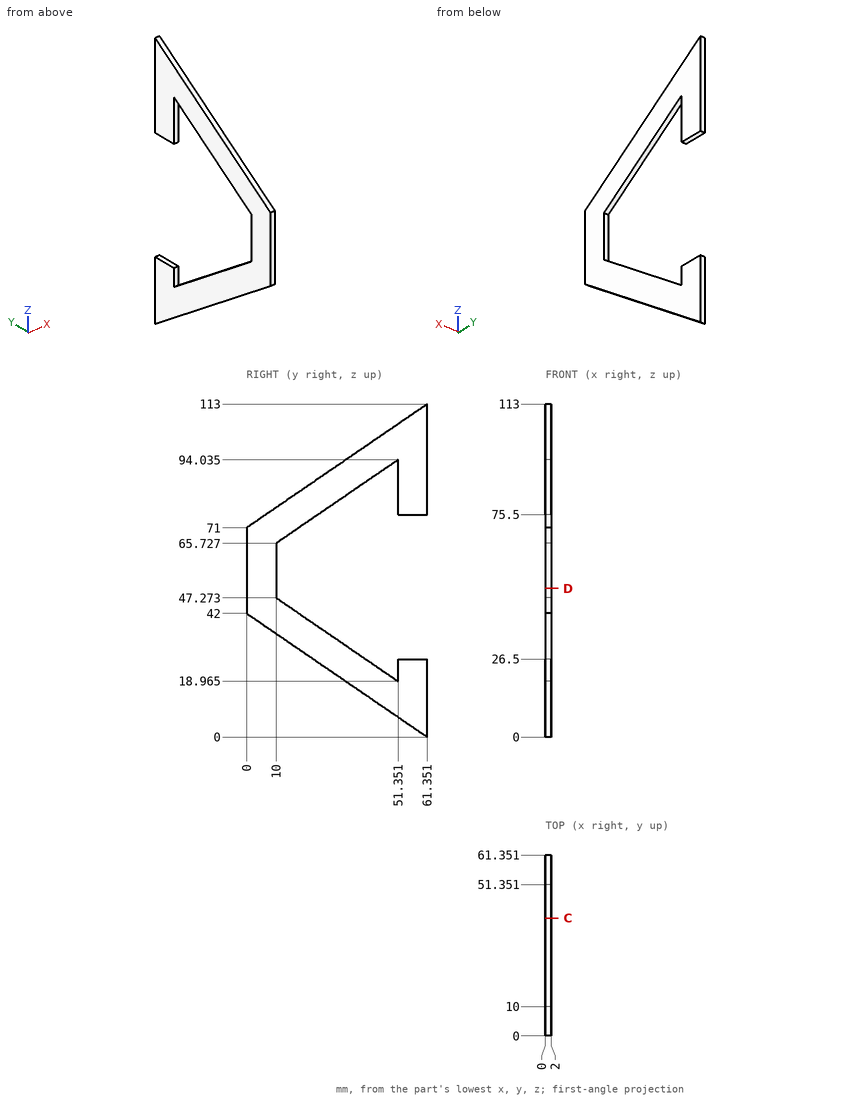
Input: dimensioned drawing with shaded views. Units: mm. Origin: part minimum x, y, z. Coordinates: 2 decimals unless noted, no trailing zeros. Order: outer loops, then holes, each group sorted by start corner. A loop starts at its lowest first (then second) coordinate and runs counter-clockwise, first axis right, second up. Notation, with made-up numbers: (65.25, 89.5) - (98.25, 89.5) arc R19 ccw to (98.25, 116.5) - close; hole circle Ø3 at (88, 13.5). An arc over 180 degrees is marked (long way). Put each result on its own line as item: value.
1. Line query: line 1 along Z through (x, y) = (1.45, 14.5) (1 decimal); line 2 along Y through (x, z) = (0.35, 63.5); line 3 along Z through (x, y) = (0.95, 17). Output: solid intervals per line, ascending.
Report:
line 1: z = 32.1 to 44.2, 68.8 to 80.9
line 2: y = 0 to 10
line 3: z = 30.36 to 42.48, 70.52 to 82.64
2. Cut plane D-D on z = 50.5. Return the cut outline in (x, y).
Report:
outline: (0, 0) - (2, 0) - (2, 10) - (0, 10) - close
3. Contact query for flat-ended pins moving along their axis: pin 1 Ø8 at (y, z) = (9, 29.5) entering from -X; pin 2 Ø1 at (x, z) = (1.5, 83) entering from -Y; pin 3 Ø0.6 at (x, z) = (1, 23.5) entering from -Y (1 decimal); pin 4 Ø1 at (x, z) = (0.5, 60) entering from +Y. Output: stop coordinate, or through.
Report:
pin 1: passes through
pin 2: stops at y = 16.8
pin 3: stops at y = 26.6
pin 4: stops at y = 10
4. Cut plane C-C on y = 40. Return the cut outline in (x, z) (1 decimal).
Report:
outline: (0, 14.6) - (2, 14.6) - (2, 26.7) - (0, 26.7) - close; (0, 86.3) - (2, 86.3) - (2, 98.4) - (0, 98.4) - close
